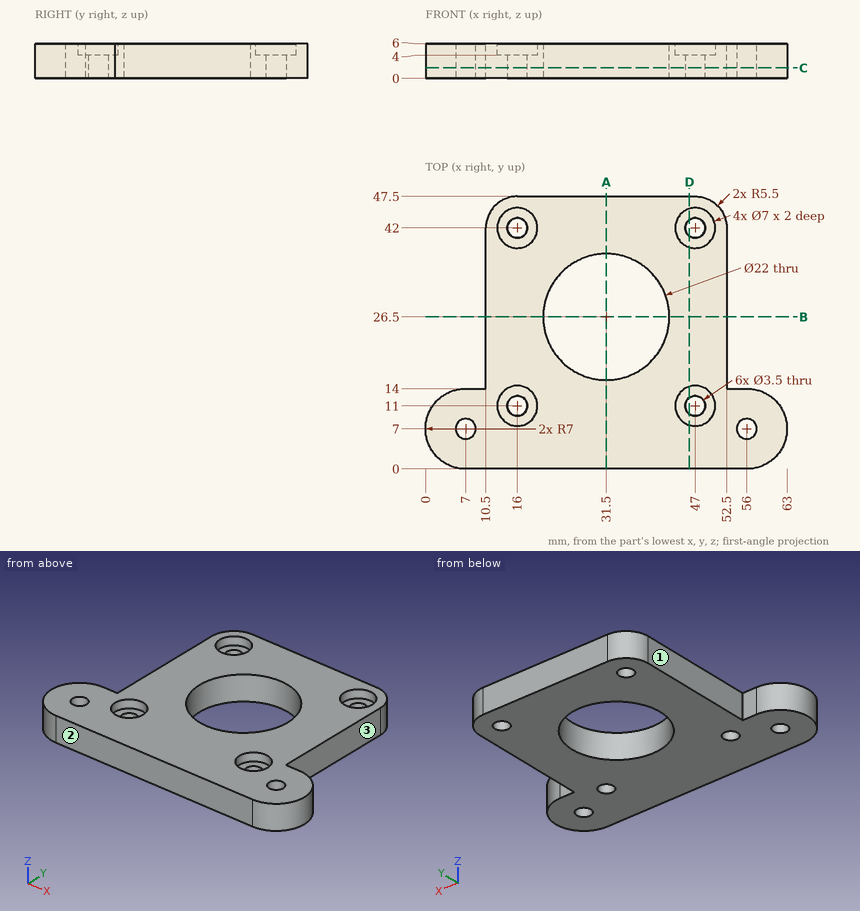
Here's the drawing with two shaded views (mm, measured from the low corner). I have some questions. A direction names the side the tool comes from. Coordinates: 2 decimals unless noted, no trailing zeros. Write each loop counter-clockwise with the first axis right and the second up, starting at its lowest first coordinate (ties: lowest second). Pieces come first, ordered by that corner, then holes. Notation, with made-up numbers: (-32, 42.25) -> (1, 42.25) arc R26 ccw to (1, 78.25) -> close; hole circle Ø4 at (-28.5, 14.5). An arc over 180 degrees is marked (long way). Use a Markdown table: item, result. Add a question column.
(1) If we section it at C-C, the plane z = 1.85: Write out the boundary of the cut face in (x, y), and give its area (3 significant figures).
(2) I'm going to push flat-ended pins straight in: P1, Ø3, axis at y = 17.5, z = 1.5, coming from the +X side; P2, Ø1.8, axis at x = 55, z = 4, coming from the +Y side; P3, Ø2, axis at x = 14.5, y = 12, coming from the +Z side; P4, Ø11, axis at x = 47, y = 42, coming from the +Z side. Where does each tip first touch, or does it pass through?
(3) If we section it at D-D, the plane x = 46: Write out the boundary of the cut face in (y, z).
(4) If we section it at B-B, the plane y = 26.5: Write out the boundary of the cut face in (x, z).
(5) For the marked faces 1, 2 and 3, which set-ups out of +Z, -Z, +X, -X, +Y, -Y let a thin tool reach every point of the face, with its end or its side?
(6) If we section it at A-A, the plane x = 31.5: Write out the boundary of the cut face in (y, z), and give its area (3 significant figures).
(7) Please list where these lines run through material, in increasing order: line 1 (Y direction, x = 16, z = 5.1); line 2 (Y direction, x = 47, z = 1.45); line 3 (X direction, y = 42, z = 1.7).
Outcome:
| question | item | result |
|---|---|---|
| 1 | outline | (7, 0) -> (56, 0) arc R7 ccw to (56, 14) -> (52.5, 14) -> (52.5, 42) arc R5.5 ccw to (47, 47.5) -> (16, 47.5) arc R5.5 ccw to (10.5, 42) -> (10.5, 14) -> (7, 14) arc R7 ccw to start; hole circle Ø3.5 at (7, 7); hole circle Ø3.5 at (16, 11); hole circle Ø3.5 at (16, 42); hole circle Ø22 at (31.5, 26.5); hole circle Ø3.5 at (47, 11); hole circle Ø3.5 at (47, 42); hole circle Ø3.5 at (56, 7) |
| 1 | area | 1,800 mm^2 |
| 2 | P1 | stops at x = 52.5 |
| 2 | P2 | stops at y = 14 |
| 2 | P3 | stops at z = 4 |
| 2 | P4 | stops at z = 6 |
| 3 | outline | (0, 0) -> (9.56, 0) -> (9.56, 4) -> (7.65, 4) -> (7.65, 6) -> (0, 6) -> close; (12.44, 0) -> (40.56, 0) -> (40.56, 4) -> (38.65, 4) -> (38.65, 6) -> (14.35, 6) -> (14.35, 4) -> (12.44, 4) -> close; (43.44, 0) -> (47.5, 0) -> (47.5, 6) -> (45.35, 6) -> (45.35, 4) -> (43.44, 4) -> close |
| 4 | outline | (10.5, 0) -> (20.5, 0) -> (20.5, 6) -> (10.5, 6) -> close; (42.5, 0) -> (52.5, 0) -> (52.5, 6) -> (42.5, 6) -> close |
| 5 | face 1 | +Z, -Z, -X, +Y |
| 5 | face 2 | +Z, -Z, +X, -X, -Y |
| 5 | face 3 | +Z, -Z, +X, +Y |
| 6 | outline | (0, 0) -> (15.5, 0) -> (15.5, 6) -> (0, 6) -> close; (37.5, 0) -> (47.5, 0) -> (47.5, 6) -> (37.5, 6) -> close |
| 6 | area | 153 mm^2 |
| 7 | line 1 | y = 0 to 7.5, 14.5 to 38.5, 45.5 to 47.5 |
| 7 | line 2 | y = 0 to 9.25, 12.75 to 40.25, 43.75 to 47.5 |
| 7 | line 3 | x = 10.5 to 14.25, 17.75 to 45.25, 48.75 to 52.5 |
